Check sheet for the drawn part. Datum: minimum x, y, z corner. Units: mm. A direction names the side the tool comes from. Round coordinates to 2 decimals unless told otherwise and drop trailing zeros. Write each loop counter-clockwise with the first axis right and the second up, starting at its lowest first coordinate (ties: lowest second). Pieces come first, ordered by that corner, then holes.
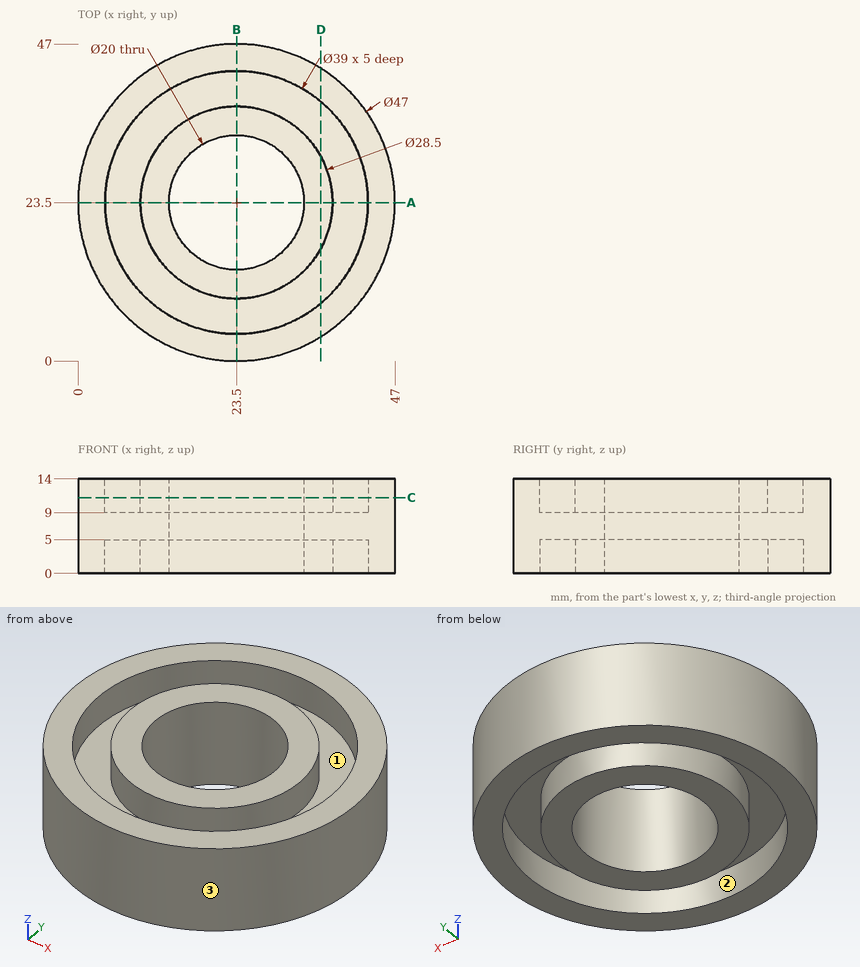
1. Go/stop test with flat-tipped pins: pin 1 (1.5 mm diameter, centred on y = 35, z = 2.5, fed in from -X); pin 2 (2 mm diameter, centred on x = 35, z = 10, fed in from -Y); pin 3 (1.5 mm diameter, centred on x = 19, z = 12, fed in from -Y). Record where each tip stops, or that it passes through.
2. Sectioned sample at C-C, the plane z = 11.25. Enter the section's corners in (x, y), plus the area to 3 significant figures.
3. Sectioned sample at A-A, the plane y = 23.5. Enter the section's corners in (x, z).
4. Set-up check for the marked faces 1, 2 and 3: record each of +Z, -Z, +X, -X, +Y, -Y from which the full face is reachable in a straight line by a thin tool's end or side.
5. Sectioned sample at D-D, the plane x = 36. Enter the section's corners in (y, z).
6. Scan lines: line 1 along Y through (x, z) = (23.5, 3.35); line 2 along Y through (x, z) = (23.5, 7.75); line 3 along Z through (x, y) = (6.5, 24). Record each from-to range of solid material in increasing order.
Computed values:
1. pin 1: stops at x = 2.6
1. pin 2: stops at y = 2.48
1. pin 3: stops at y = 0.3
2. outline: circle Ø47 at (23.5, 23.5); circle Ø28.5 at (23.5, 23.5); hole circle Ø39 at (23.5, 23.5); hole circle Ø20 at (23.5, 23.5)
2. area: 864 mm2
3. outline: (0, 0) - (4, 0) - (4, 5) - (9.25, 5) - (9.25, 0) - (13.5, 0) - (13.5, 14) - (9.25, 14) - (9.25, 9) - (4, 9) - (4, 14) - (0, 14) - close; (33.5, 0) - (37.75, 0) - (37.75, 5) - (43, 5) - (43, 0) - (47, 0) - (47, 14) - (43, 14) - (43, 9) - (37.75, 9) - (37.75, 14) - (33.5, 14) - close
4. face 1: +Z
4. face 2: -Z
4. face 3: +Z, -Z
5. outline: (3.6, 0) - (8.53, 0) - (8.53, 5) - (16.66, 5) - (16.66, 0) - (30.34, 0) - (30.34, 5) - (38.47, 5) - (38.47, 0) - (43.4, 0) - (43.4, 14) - (38.47, 14) - (38.47, 9) - (30.34, 9) - (30.34, 14) - (16.66, 14) - (16.66, 9) - (8.53, 9) - (8.53, 14) - (3.6, 14) - close
6. line 1: y = 0 to 4, 9.25 to 13.5, 33.5 to 37.75, 43 to 47
6. line 2: y = 0 to 13.5, 33.5 to 47
6. line 3: z = 5 to 9
